from build123d import *

# Parameters (mm, degrees)
F0_R     = 6.35
F1_DEPTH = 15.875
F2_DEPTH = 25.4
F3_W     = 19.05
F3_H     = 19.05
F4_DEPTH = 618.600804


with BuildPart() as f1:
    # F0 (on Front) → F1 (new body)
    with BuildSketch(Plane.XZ):
        Polygon((301.713325, -54.802002), (-291.486479, -54.802002), (-304.186479, -54.802002), (-304.186479, -80.202002), (-291.486479, -80.202002), (301.713325, -80.202002), (314.413325, -80.202002), (314.413325, -54.802002), align=None)
        with Locations((-291.486479, -67.502002)):
            Circle(F0_R, mode=Mode.SUBTRACT)
        with Locations((301.713325, -67.502002)):
            Circle(F0_R, mode=Mode.SUBTRACT)
    extrude(amount=F1_DEPTH)

    # F0 (on Front) → F2 (join)
    with BuildSketch(Plane.XZ):
        Polygon((301.713325, -54.802002), (-291.486479, -54.802002), (-304.186479, -54.802002), (-304.186479, -80.202002), (-291.486479, -80.202002), (301.713325, -80.202002), (314.413325, -80.202002), (314.413325, -54.802002), align=None)
        with Locations((-291.486479, -67.502002)):
            Circle(F0_R, mode=Mode.SUBTRACT)
        with Locations((301.713325, -67.502002)):
            Circle(F0_R, mode=Mode.SUBTRACT)
    extrude(amount=F2_DEPTH)

    # F3 (on face) → F4 (cut, through all)
    with BuildSketch(Plane.YZ.offset(314.413325)):
        with Locations((-12.7, -67.502002)):
            Rectangle(F3_W, F3_H)
    extrude(amount=-F4_DEPTH, mode=Mode.SUBTRACT)


solid = f1.part
Verification items for the finished model (mm, model axes). A direction names the side the tool comes from. Coordinates: 2 decimals unless noted, no trailing zeros. Loops run counter-clockwise (first coordinate to the right, second up) from the corner with the lowest first, then second, coordinate; pieces in that order, holes last. Notation, with made-up numbers: (72.25, 79.5) -> (126.25, 79.5) arc R25 ccw to (126.25, 113.5) -> close; hole circle Ø10 at (-35, 36). An arc over 180 degrees is marked (long way). Answer as a JSON object with one key per item and string values. Group by question number.
Item 1: Tool access check on faces 4 (the flat face through (9, -13, -57.977)), 5 (the flat face through (1, 0, -67)). Record the directions out of +Z, -Z, +X, -X, +Y, -Y that give a thin tool (end or side, any length) a straight path to the whole face; none if there is none.
Item 2: Mould release check, pull along X, two halves, no side actions. Record for faces 1 (the flat face through (314.413, -13, -79)), 2 (the cylindrical face through (-288.556, -23.79, -73.136)), 3 (the flat face through (1, -25.4, -67)): +X half, -X half, draft (parallel to the pull), parting line (faces both ways), or undercut.
Item 3: Sectioned sample at B-B on x = -36. Record the boundary of the cut face in (y, z) (3 decimals).
Item 4: Sectioned sample at A-A on y = -10.5. Record the boundary of the cut face in (x, z), plus the area to 3 significant figures.
Item 5: Scan lines: probe 1 along Y at (x, z) = (261, -68.25) (3 decimals); probe 2 along Z at (x, y) = (223.5, -8). Record each from-to range of solid material in increasing order.
Evaluation:
{
 "1": {"face 4": "+X, -X", "face 5": "+Z, -Z, +X, -X, +Y"},
 "2": {"face 1": "+X half", "face 2": "undercut", "face 3": "draft"},
 "3": {"outline": "(-25.4, -80.202) -> (0, -80.202) -> (0, -54.802) -> (-25.4, -54.802) -> close; hole (-22.225, -77.027) -> (-3.175, -77.027) -> (-3.175, -57.977) -> (-22.225, -57.977) -> close"},
 "4": {"outline": "(-304.19, -80.2) -> (314.41, -80.2) -> (314.41, -77.03) -> (-304.19, -77.03) -> close; (-304.19, -57.98) -> (314.41, -57.98) -> (314.41, -54.8) -> (-304.19, -54.8) -> close", "area": "3,930 mm²"},
 "5": {"probe 1": "y = -25.4 to -22.225, -3.175 to 0", "probe 2": "z = -80.2 to -77.03, -57.98 to -54.8"}
}
